Part model, mm, in its own coordinate system. Give positions to 0.01 mm unless a question says otherwise; leave off trailing zeros. Order: outer loops, then holes, each group sorted by start corner. A loop starts at its lowest first (then second) coordinate and runs counter-clockwise, first axis right, second up. Notation, with made-up numbers: M 34,38.25 L 53,38.25 A29 ccw 53,63.25 Z; hole C 30.25,-21.75 d6. An arc over 180 degrees is marked long. Return JSON: item names as keys, results as strings.
from build123d import *

# Parameters (mm, degrees)
SKETCH_1_W      = 30
SKETCH_1_H      = 280
EXTRUDE_1_DEPTH = 5
SKETCH_2_W      = 13
SKETCH_2_H      = 280
EXTRUDE_2_DEPTH = 20


with BuildPart() as part:
    # 草图1 → 凸台-拉伸1 (new body)
    with BuildSketch(Plane(origin=(0, 0, 0), x_dir=(1, 0, 0), z_dir=(0, 1, 0))):
        with Locations((15, -93.34585106)):
            Rectangle(SKETCH_1_W, SKETCH_1_H)
    extrude(amount=-EXTRUDE_1_DEPTH)

    # 草图2 → 凸台-拉伸2 (add)
    with BuildSketch(Plane(origin=(0, 0, 0), x_dir=(1, 0, 0), z_dir=(0, 1, 0))):
        with Locations((6.5, -93.34585106)):
            Rectangle(SKETCH_2_W, SKETCH_2_H)
        with Locations((23.5, -93.34585106)):
            Rectangle(SKETCH_2_W, SKETCH_2_H)
    extrude(amount=EXTRUDE_2_DEPTH)


solid = part.part
Q1. Band-saw the part on B-B (y = 13). Give the cut face in (x, z), then the cut area to 3 significant figures.
Established:
{"outline": "M 0,-46.65 L 13,-46.65 L 13,233.35 L 0,233.35 Z; M 17,-46.65 L 30,-46.65 L 30,233.35 L 17,233.35 Z", "area": "7,280 mm²"}
Q2. Probe line 1 along X through (y, z) = (14.5, 70); line 2 along Y through (x, z) = (14.5, 68.5). List the from-to ranges inside material, lowest first.
Established:
{"line 1": "x = 0 to 13, 17 to 30", "line 2": "y = -5 to 0"}
Q3. Two-plate mould, pull along X, no slides. Class faces 1 (the flat face through (11, 7, 233.346)), 2 (the flat face through (13, 10, 95)), 3 (the flat face through (0, 7, 95)), 4 (the flat face through (17, 10, 95)): +X half, -X half, draft (parallel to the pull), parting line (faces both ways), or undercut.
Established:
{"face 1": "draft", "face 2": "undercut", "face 3": "-X half", "face 4": "undercut"}
Q4. Band-saw the part on A-A (z = 47). Give the cut face in (x, y), then the cut area to 3 significant figures.
Established:
{"outline": "M 0,-5 L 30,-5 L 30,20 L 17,20 L 17,0 L 13,0 L 13,20 L 0,20 Z", "area": "670 mm²"}
